Job drawing, mm, ordinate dimensions from the low corner. One solid piece. A direction names the side the tool comes from. Give positions to 0.01 mm unless a question says otherwise; leave off trailing zeros. Loops run counter-clockwise (first coordinate to the right, second up) from the corner with the lowest first, then second, coordinate; pieces in that order, holes last. Notation, with made-up numbers: M 53,-3.5 L 112,-3.5 A17 cw 112,16.5 Z; hole C 44.5,-7.75 d8. An arc over 180 degrees is marked long. Put each result on its own line as item: value.
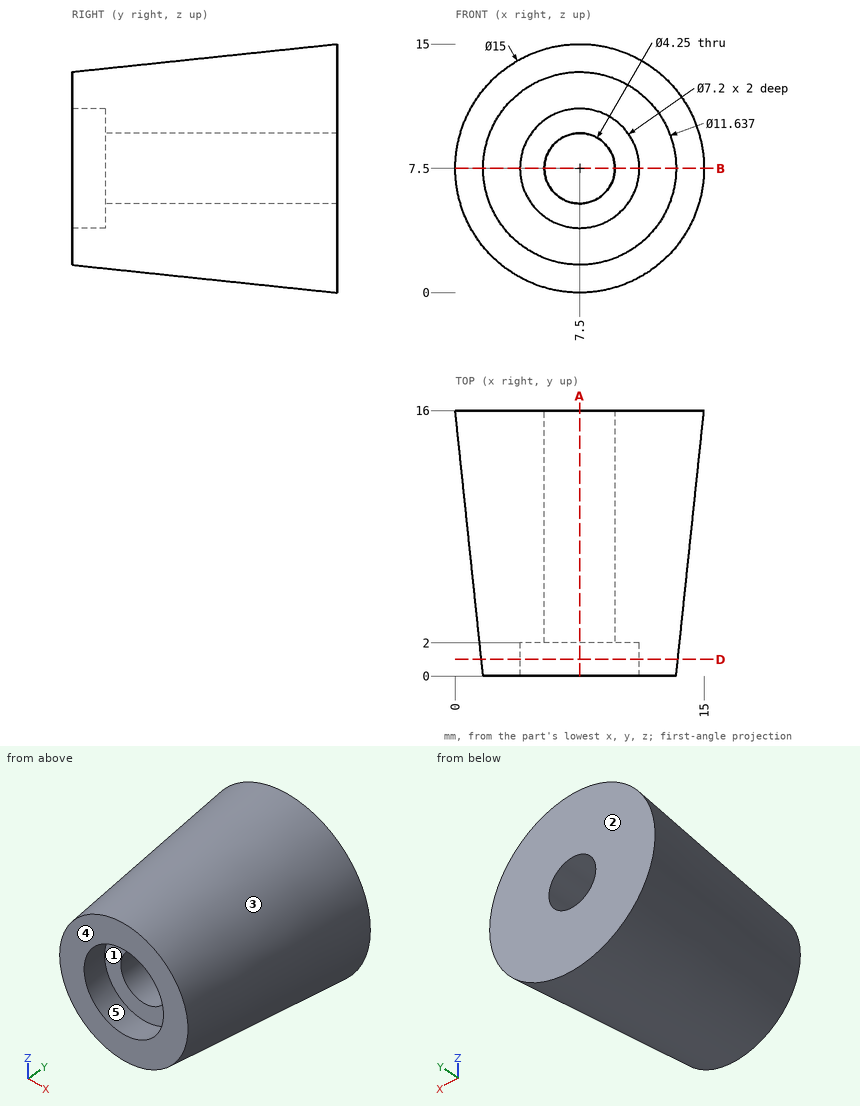
Q1. Slice it at D-D (y = 1). List the corners of the cut face in (x, z).
Here are the results:
outline: C 7.5,7.5 d11.85; hole C 7.5,7.5 d7.2
Q2. Drop flat-ended pins along their axis: pin 1 Ø8 at (x, y) = (5, 5.5) entering from +Z; pin 2 Ø8 at (x, z) = (8.5, 8) entering from -Y; pin 3 Ø5 at (y, z) = (11.5, 12) entering from +X; pin 4 Ø6 at (x, y) = (5, 13.5) entering from +Z. Give the stop position or say it passes through.
Here are the results:
pin 1: z = 14.24
pin 2: y = 0
pin 3: x = 14.28
pin 4: z = 14.96
Q3. Slice it at A-A (x = 7.5). List the corners of the cut face in (y, z) (1 decimal).
Here are the results:
outline: M 0,1.7 L 16,0 L 16,5.4 L 2,5.4 L 2,3.9 L 0,3.9 Z; M 0,11.1 L 2,11.1 L 2,9.6 L 16,9.6 L 16,15 L 0,13.3 Z
Q4. Mould opens along X. For the marked faces 3, 4 and 5 say: pulls with the +X half, pulls with the -X half, needs draft (parallel to the pull), parting line crosses it, or undercut.
Here are the results:
face 3: parting line crosses it
face 4: needs draft
face 5: undercut
Q5. Tool access for the marked faces 1 and 2: list every direction of +Z, -Z, +X, -X, +Y, -Y with a clear straight run to the whole face (end or side of a thin tool).
Here are the results:
face 1: -Y
face 2: +Z, -Z, +X, -X, +Y
Q6. Probe line 1 (Y direction, x = 6.25, z = 10.75); line 2 (X direction, y = 3, z = 7.25); line 3 (Z direction, x = 7.5, y = 9) (1 decimal). List the from-to ranges inside material, lowest first. Write a range as from..to.
Here are the results:
line 1: 2..16
line 2: 1.37..5.39, 9.61..13.63
line 3: 0.7..5.4, 9.6..14.3
Q7. Slice it at B-B (z = 7.5). List the corners of the cut face in (x, y) (1 decimal), and give its area (3 significant figures).
Here are the results:
outline: M 0,16 L 1.7,0 L 3.9,0 L 3.9,2 L 5.4,2 L 5.4,16 Z; M 9.6,2 L 11.1,2 L 11.1,0 L 13.3,0 L 15,16 L 9.6,16 Z
area: 139 mm²
